```python
from build123d import *

# Parameters (mm, degrees)
SKETCH_W     = 12
SKETCH_H     = 14
SKETCH_R     = 2.5
PAD_DEPTH    = 3
SKETCH001_W  = 2
SKETCH001_H  = 14
PAD001_DEPTH = 16
SKETCH002_W  = 14
SKETCH002_H  = 3
PAD008_DEPTH = 10
SKETCH004_W  = 14
SKETCH004_H  = 3
PAD004_DEPTH = 8
SKETCH003_W  = 34
SKETCH003_H  = 3
PAD009_DEPTH = 8
SKETCH006_R  = 2
POCKET_DEPTH = 19.001
PAD005_DEPTH = 3
SKETCH008_W  = 20
SKETCH008_H  = 19
PAD006_DEPTH = 3
SKETCH009_W  = 2
SKETCH009_H  = 19
PAD007_DEPTH = 2
FILLET_R     = 1.5
FILLET001_R  = 1.5
FILLET002_R  = 1
FILLET003_R  = 1
FILLET004_R  = 0.5
FILLET005_R  = 0.5


with BuildPart() as part:
    # Sketch → Pad (new body)
    with BuildSketch(Plane.XY):
        with Locations((1, 0)):
            Rectangle(SKETCH_W, SKETCH_H)
        Circle(SKETCH_R, mode=Mode.SUBTRACT)
    extrude(amount=PAD_DEPTH)

    # Sketch001 (on Face7 of Pad) → Pad001 (join)
    with BuildSketch(Plane.XY.offset(3)):
        with Locations((6, 0)):
            Rectangle(SKETCH001_W, SKETCH001_H)
    extrude(amount=PAD001_DEPTH)

    # Sketch002 (on Face10 of Pad001) → Pad008 (join)
    with BuildSketch(Plane(origin=(5, 0, 0), x_dir=(0, -1, 0), z_dir=(-1, 0, 0))):
        with Locations((0, 17.5)):
            Rectangle(SKETCH002_W, SKETCH002_H)
    extrude(amount=PAD008_DEPTH)

    # Sketch004 → Pad004 (join)
    with BuildSketch(Plane(origin=(-5, 0, 0), x_dir=(0, -1, 0), z_dir=(-1, 0, 0))):
        with Locations((0, 1.5)):
            Rectangle(SKETCH004_W, SKETCH004_H)
    extrude(amount=PAD004_DEPTH)

    # Sketch003 → Pad009 (join)
    with BuildSketch(Plane(origin=(-5, 0, 0), x_dir=(0, -1, 0), z_dir=(-1, 0, 0))):
        with Locations((-10, 17.5)):
            Rectangle(SKETCH003_W, SKETCH003_H)
    extrude(amount=PAD009_DEPTH)

    # Sketch006 → Pocket (cut, through all)
    with BuildSketch(Plane.XY.offset(19)):
        with Locations((-9, 22)):
            Circle(SKETCH006_R)
        with Locations((-9, 12)):
            Circle(SKETCH006_R)
    extrude(amount=-POCKET_DEPTH, mode=Mode.SUBTRACT)

    # Sketch007 (on Face26 of Pocket) → Pad005 (join)
    with BuildSketch(Plane(origin=(-13, 0, 0), x_dir=(0, -1, 0), z_dir=(-1, 0, 0))):
        Polygon((-27, 19), (7, 19), (7, 0), (-7, 0), (-27, 16), align=None)
    extrude(amount=PAD005_DEPTH)

    # Sketch008 (on Face10 of Pad005) → Pad006 (join)
    with BuildSketch(Plane.XZ.offset(7)):
        with Locations((-6, 9.5)):
            Rectangle(SKETCH008_W, SKETCH008_H)
    extrude(amount=PAD006_DEPTH)

    # Sketch009 (on Face15 of Pad006) → Pad007 (join)
    with BuildSketch(Plane(origin=(5, 0, 0), x_dir=(0, -1, 0), z_dir=(-1, 0, 0))):
        with Locations((6, 9.5)):
            Rectangle(SKETCH009_W, SKETCH009_H)
    extrude(amount=PAD007_DEPTH)

    # Fillet
    fillet_edges = [part.edges().sort_by_distance(p)[0] for p in [
        (7, 0, 0),
    ]]
    fillet(fillet_edges, radius=FILLET_R)

    # Fillet001
    fillet001_edges = [part.edges().sort_by_distance(p)[0] for p in [
        (-16, 0, 0),
    ]]
    fillet(fillet001_edges, radius=FILLET001_R)

    # Fillet002
    fillet002_edges = [part.edges().sort_by_distance(p)[0] for p in [
        (7, 0, 19),
    ]]
    fillet(fillet002_edges, radius=FILLET002_R)

    # Fillet003
    fillet003_edges = [part.edges().sort_by_distance(p)[0] for p in [
        (-16, 10, 19),
    ]]
    fillet(fillet003_edges, radius=FILLET003_R)

    # Fillet004
    fillet004_edges = [part.edges().sort_by_distance(p)[0] for p in [
        (-5, 17, 19),
    ]]
    fillet(fillet004_edges, radius=FILLET004_R)

    # Fillet005
    fillet005_edges = [part.edges().sort_by_distance(p)[0] for p in [
        (-14, 27, 19),
        (-9.25, 27, 19),
    ]]
    fillet(fillet005_edges, radius=FILLET005_R)


solid = part.part
```
Here's how the part is built. I have some questions about the finished solid (model axes, mm). A direction names the side the tool comes from. Round coordinates to 2 decimals unless told otherwise and drop trailing zeros. Order: outer loops, then holes, each group sorted by start corner. A loop starts at its lowest first (then second) coordinate and runs counter-clockwise, first axis right, second up. Notation, with made-up numbers: M -6,86 L 23,86 A34 ccw 23,124 Z; hole C 69.5,42 d10. An arc over 180 degrees is marked long. Answer as CSV lines item,"result".
Item 1: Imagine slicing it at A-A on y = 22. List the corners of the cut face in (x, z) for me, and give its area (3 significant figures).
From the geometry:
outline,"M -16,12 L -13,12 L -13,16 L -11,16 L -11,19 L -15,19 A1 ccw -16,18 Z; M -7,16 L -5,16 L -5,18.5 A0.5 ccw -5.5,19 L -7,19 Z"
area,"32.7 mm2"
Item 2: We'd pull the mould along Y, two halves only. Please class faces 4 (the cylindrical face through (6.55, 0.1, 0.43)), 5 (the cylindrical face through (-9, 14, 18)), 6 (the flat face through (5.2, 7, 6.6)), 7 (the cylindrical face through (-0.54, -2.44, 1.48)): +Y half, -Y half, draft (parallel to the pull), parting line (faces both ways), or undercut.
From the geometry:
face 4,"draft"
face 5,"undercut"
face 6,"+Y half"
face 7,"undercut"
Item 3: Imagine slicing it at C-C on x = -4.25. List the corners of the cut face in (y, z) for me, and give its area (3 significant figures).
From the geometry:
outline,"M -10,0 L 7,0 L 7,3 L -7,3 L -7,16 L 7,16 L 7,19 L -10,19 Z"
area,"141 mm2"
Item 4: Which directions (+Z, -Z, +X, -X, +Y, -Y) give clear straight access to the entire face, cutting with the end or side of a thin tool? Please do faces 1 (the flat face through (-5, 17, 17)), 2 (the flat face through (6, -7, 10)), 3 (the flat face through (-6, 6, 16)).
From the geometry:
face 1,"+Z, -Z, +X, +Y"
face 2,"+Z, -Z, +X, -Y"
face 3,"+Y"
Item 5: For pin 1 (2.5 mm diameter, centred on x = -9, y = 22, fed in from +Z); pin 2 (9.5 mm diameter, centred on x = -4.5, z = 5.5, fed in from +Y); pin 3 (0.8 mm diameter, centred on y = 13.5, z = 18, fed in from +X); pin 4 (1 mm diameter, centred on x = 3.5, z = 12, fed in from +Y), each with a flat end and sliding along its axis, tell me the tip position at first contact or that it passes through.
From the geometry:
pin 1,"through"
pin 2,"y = 7"
pin 3,"x = -5"
pin 4,"y = -5"
Item 6: Please list where these lines run through material, in increasing order: L1, parallel to Y at x = -9, z = 17.5; L2, parallel to Z at x = -7.25, y = 6; L3, parallel to Z at x = -11.25, y = 15. Write a range as [from, to].
From the geometry:
L1,"[-10, 10], [14, 20], [24, 27]"
L2,"[0, 3], [16, 19]"
L3,"[16, 19]"
Item 7: Imagine slicing it at B-B on x = 1.5. List the corners of the cut face in (y, z) for me, and give its area (3 significant figures).
From the geometry:
outline,"M -10,0 L -2,0 L -2,3 L -7,3 L -7,16 L 7,16 L 7,19 L -10,19 Z; M 2,0 L 7,0 L 7,3 L 2,3 Z"
area,"129 mm2"
Item 8: Imagine slicing it at D-D on y = 5. List the corners of the cut face in (x, z) for me.
From the geometry:
outline,"M -16,1.5 A1.5 ccw -14.5,0 L 5.5,0 A1.5 ccw 7,1.5 L 7,18 A1 ccw 6,19 L -15,19 A1 ccw -16,18 Z; hole M -13,3 L 5,3 L 5,16 L -13,16 Z"
